```python
from build123d import *
from OCP.BRepFilletAPI import BRepFilletAPI_MakeChamfer

# Parameters (mm, degrees)
SKETCH1_W           = 50
SKETCH1_H           = 30
SKETCH1_R           = 2.5
BOSS_EXTRUDE1_DEPTH = 15
SKETCH2_W           = 15
SKETCH2_H           = 30
CUT_EXTRUDE1_DEPTH  = 10
CHAMFER1_SIZE       = 0.75
CHAMFER1_SIZE2      = 1.299038106
SHELL1_START        = 2
SHELL1_OUTLINE_W    = 15.5
SHELL1_OUTLINE_H    = 26
SHELL1_OUTLINE_R    = 4.5
SHELL1_DEPTH        = 13
SHELL1_2_OUTLINE_W  = 15
SHELL1_2_OUTLINE_H  = 26
SHELL1_2_DEPTH      = 1
SKETCH3_R           = 3.5
CUT_EXTRUDE2_DEPTH  = 5
SKETCH4_R           = 3.5
CUT_EXTRUDE3_DEPTH  = 5
SKETCH5_R           = 3.5
CUT_EXTRUDE4_DEPTH  = 5
SKETCH6_R           = 3.5
CUT_EXTRUDE5_DEPTH  = 5
CHAMFER2_SIZE       = 1


# Read off the part's stored shape, not the designer's step: Shell1
with BuildPart() as part:
    # Sketch1 → Boss-Extrude1 (new body)
    with BuildSketch(Plane(origin=(0, 0, 0), x_dir=(1, 0, 0), z_dir=(0, 1, 0))):
        Rectangle(SKETCH1_W, SKETCH1_H)
        with Locations(Location((-17.5, 7.5, 0), (0, 0, 270))):
            Circle(SKETCH1_R, mode=Mode.SUBTRACT)
        with Locations(Location((17.5, 7.5, 0), (0, 0, 90))):
            Circle(SKETCH1_R, mode=Mode.SUBTRACT)
        with Locations(Location((17.5, -7.5, 0), (0, 0, 270))):
            Circle(SKETCH1_R, mode=Mode.SUBTRACT)
        with Locations(Location((-17.5, -7.5, 0), (0, 0, 90))):
            Circle(SKETCH1_R, mode=Mode.SUBTRACT)
    extrude(amount=BOSS_EXTRUDE1_DEPTH)

    # Sketch2 → Cut-Extrude1 (cut)
    with BuildSketch(Plane(origin=(0, 15, 0), x_dir=(1, 0, 0), z_dir=(0, 1, 0))):
        Rectangle(SKETCH2_W, SKETCH2_H)
    extrude(amount=-CUT_EXTRUDE1_DEPTH, mode=Mode.SUBTRACT)

    # Chamfer1: one chamfer whose edges measure the first distance from different faces: ONE call of the kernel's chamfer builder (chamfer() names one face for all edges)
    chamfer1_edges_1 = [part.edges().sort_by_distance(p)[0] for p in [
        (-17.5, 0, -10),
    ]]
    chamfer1_side_1 = [part.faces().sort_by_distance(p)[0] for p in [
        (-17.5, 7.5, -10),
    ]]
    chamfer1_edges_2 = [part.edges().sort_by_distance(p)[0] for p in [
        (17.5, 0, -5),
    ]]
    chamfer1_side_2 = [part.faces().sort_by_distance(p)[0] for p in [
        (17.5, 7.5, -5),
    ]]
    chamfer1_edges_3 = [part.edges().sort_by_distance(p)[0] for p in [
        (17.5, 0, 5),
    ]]
    chamfer1_side_3 = [part.faces().sort_by_distance(p)[0] for p in [
        (17.5, 7.5, 5),
    ]]
    chamfer1_edges_4 = [part.edges().sort_by_distance(p)[0] for p in [
        (-17.5, 0, 10),
    ]]
    chamfer1_side_4 = [part.faces().sort_by_distance(p)[0] for p in [
        (-17.5, 7.5, 10),
    ]]
    chamfer1 = BRepFilletAPI_MakeChamfer(part.part.solid().wrapped)
    for e in chamfer1_edges_1:
        chamfer1.Add(CHAMFER1_SIZE, CHAMFER1_SIZE2, e.wrapped, chamfer1_side_1[0].wrapped)  # the first distance lies on this face
    for e in chamfer1_edges_2:
        chamfer1.Add(CHAMFER1_SIZE, CHAMFER1_SIZE2, e.wrapped, chamfer1_side_2[0].wrapped)  # the first distance lies on this face
    for e in chamfer1_edges_3:
        chamfer1.Add(CHAMFER1_SIZE, CHAMFER1_SIZE2, e.wrapped, chamfer1_side_3[0].wrapped)  # the first distance lies on this face
    for e in chamfer1_edges_4:
        chamfer1.Add(CHAMFER1_SIZE, CHAMFER1_SIZE2, e.wrapped, chamfer1_side_4[0].wrapped)  # the first distance lies on this face
    add(Compound.cast(chamfer1.Shape()), mode=Mode.REPLACE)

    # Shell1 outline → Shell1 (cut)
    # profile 1 of 2: a face of its own
    with BuildSketch(Plane(origin=(0, 0, 0), x_dir=(1, 0, 0), z_dir=(0, 1, 0)).offset(SHELL1_START)):
        with Locations((-15.25, 0)):
            Rectangle(SHELL1_OUTLINE_W, SHELL1_OUTLINE_H)
        with Locations((-17.5, -7.5)):
            Circle(SHELL1_OUTLINE_R, mode=Mode.SUBTRACT)
        with Locations((-17.5, 7.5)):
            Circle(SHELL1_OUTLINE_R, mode=Mode.SUBTRACT)
    # profile 2 of 2: a face of its own
    with BuildSketch(Plane(origin=(0, 0, 0), x_dir=(1, 0, 0), z_dir=(0, 1, 0)).offset(SHELL1_START)):
        with Locations((15.25, 0)):
            Rectangle(SHELL1_OUTLINE_W, SHELL1_OUTLINE_H)
        with Locations((17.5, -7.5)):
            Circle(SHELL1_OUTLINE_R, mode=Mode.SUBTRACT)
        with Locations((17.5, 7.5)):
            Circle(SHELL1_OUTLINE_R, mode=Mode.SUBTRACT)
    extrude(amount=SHELL1_DEPTH, mode=Mode.SUBTRACT)

    # Shell1 2 outline → Shell1 2 (cut)
    with BuildSketch(Plane(origin=(0, 0, 0), x_dir=(1, 0, 0), z_dir=(0, 1, 0)).offset(SHELL1_START)):
        Rectangle(SHELL1_2_OUTLINE_W, SHELL1_2_OUTLINE_H)
    extrude(amount=SHELL1_2_DEPTH, mode=Mode.SUBTRACT)

    # Sketch3 → Cut-Extrude2 (cut)
    with BuildSketch(Plane(origin=(0, 15, 0), x_dir=(1, 0, 0), z_dir=(0, 1, 0))):
        with Locations(Location((-17.5, -7.5, 0), (0, 0, 270))):
            Circle(SKETCH3_R)
    extrude(amount=-CUT_EXTRUDE2_DEPTH, mode=Mode.SUBTRACT)

    # Sketch4 → Cut-Extrude3 (cut)
    with BuildSketch(Plane(origin=(0, 15, 0), x_dir=(1, 0, 0), z_dir=(0, 1, 0))):
        with Locations(Location((-17.5, 7.5, 0), (0, 0, 270))):
            Circle(SKETCH4_R)
    extrude(amount=-CUT_EXTRUDE3_DEPTH, mode=Mode.SUBTRACT)

    # Sketch5 → Cut-Extrude4 (cut)
    with BuildSketch(Plane(origin=(0, 15, 0), x_dir=(1, 0, 0), z_dir=(0, 1, 0))):
        with Locations(Location((17.5, 7.5, 0), (0, 0, 270))):
            Circle(SKETCH5_R)
    extrude(amount=-CUT_EXTRUDE4_DEPTH, mode=Mode.SUBTRACT)

    # Sketch6 → Cut-Extrude5 (cut)
    with BuildSketch(Plane(origin=(0, 15, 0), x_dir=(1, 0, 0), z_dir=(0, 1, 0))):
        with Locations(Location((17.5, -7.5, 0), (0, 0, 270))):
            Circle(SKETCH6_R)
    extrude(amount=-CUT_EXTRUDE5_DEPTH, mode=Mode.SUBTRACT)

    # Chamfer2
    chamfer2_edges = [part.edges().sort_by_distance(p)[0] for p in [
        (0, 0, -15),
        (25, 0, 0),
        (0, 0, 15),
        (-25, 0, 0),
    ]]
    chamfer(chamfer2_edges, length=CHAMFER2_SIZE)


solid = part.part
```
Read the model definition and answer for the solid it produces. Units are mm, in the model's axes. A direction names the side the tool comes from. Give positions to 0.01 mm unless a question says otherwise; leave off trailing zeros. Order: outer loops, then holes, each group sorted by start corner. A loop starts at its lowest first (then second) coordinate and runs counter-clockwise, first axis right, second up.
(1) Given pin 1 (5.5 mm diameter, centred on x = -17.5, z = -7.5, fed in from -Y); pin 2 (5.5 mm diameter, centred on x = 16, z = -6, fed in from +Y); pin 3 (6.5 mm diameter, centred on x = 17.5, z = 7.5, fed in from +Y); pin 4 (3 mm diameter, centred on x = 17.5, z = -7.5, fed in from +Y), each flat-ended and moving along its own axis, determine where each tip first touches the part or whether it passes through.
(2) For a pull along Z with two mould halves and no side action, classify faces 1 (the cylindrical face through (19.61, 5.31, 8.84)), 2 (the flat face through (0, 5, 0)) as released by +Z, released by -Z, zero draft, split by the parting line, or undercut.
(3) Straight lines are drawn through the part: L1, parallel to X at y = 12.95, z = 7.5; L2, parallel to X at y = 6, z = 7.5; L3, parallel to Z at x = 17.5, y = 7.25. For each, find the intervals that lie inside material, in ascending order.
(4) For faces 3 (the flat face through (25, 8, 0)), 4 (the flat face through (-7.5, 10, -14)), 5 (the cylindrical face through (-15.135, 12.535, -10.08)), determine the directions among +Z, -Z, +X, -X, +Y, -Y from which every point of the face is accessible in a straight line to the end or side of a thin tool.
(5) Find section B-B (x = 5.5). Give the vertices of the cut face in (y, z), plus the area to 3 significant figures.
(6) Find section D-D (y = 1.5). Give the vertices of the cut face in (x, z), plus the area to 3 significant figures.
(7) Find section A-A (y = 7.25). Give the number of separate pieces and of enclosed holes in the cut face, plus the area to 3 significant figures.
Result sheet:
1. pin 1: stops at y = 0.61
1. pin 2: stops at y = 15
1. pin 3: stops at y = 10
1. pin 4: passes through
2. face 1: undercut
2. face 2: zero draft
3. L1: x = -25 to -23, -22 to -21, -14 to -13, 13 to 14, 21 to 22, 23 to 25
3. L2: x = -25 to -23, -22 to -20, -15 to -13, 13 to 15, 20 to 22, 23 to 25
3. L3: z = -15 to -13, -12 to -10, -5 to -3, 3 to 5, 10 to 12, 13 to 15
4. face 3: +Z, -Z, +X, +Y, -Y
4. face 4: +Z, -Z, +Y
4. face 5: +Y
5. outline: (0, -14) - (1, -15) - (5, -15) - (5, 15) - (1, 15) - (0, 14) - close; hole (2, -13) - (3, -13) - (3, 13) - (2, 13) - close
5. area: 123 mm2
6. outline: (-25, -15) - (25, -15) - (25, 15) - (-25, 15) - close; hole circle Ø5 at (-17.5, -7.5); hole circle Ø5 at (-17.5, 7.5); hole circle Ø5 at (17.5, -7.5); hole circle Ø5 at (17.5, 7.5)
6. area: 1,420 mm2
7. separate pieces: 6
7. enclosed holes: 4
7. area: 420 mm2
